from build123d import *

# Parameters (mm, degrees)
F1_DEPTH       = 40
F3_D           = 6.6
F3_CSINK_D     = 13.44
F3_CSINK_ANGLE = 90


# Not quite as in the source:
# - a feature names something its author has since deleted; it is built from what else it names


with BuildPart() as f1:
    # F0 (on Front) → F1 (new body)
    with BuildSketch(Plane.XZ):
        Polygon((52.3067873225, 0), (0, 0), (0, -17), align=None)
    extrude(amount=F1_DEPTH)

    # F3 (through all)
    with Locations(Plane(origin=(4.997243483, 0, -15.3758677686), x_dir=(0.9510324968, 0, 0.3090909091), z_dir=(0.3090909091, 0, -0.9510324968))):
        with Locations((9.5479916781, 20), (30.6618269533, 20)):
            CounterSinkHole(F3_D / 2, F3_CSINK_D / 2, counter_sink_angle=F3_CSINK_ANGLE)


solid = f1.part
The model under review builds one solid part; all positions refer to its coordinate system, in mm. Give positions to 0.01 mm unless a question says otherwise; leave off trailing zeros. Order: outer loops, then holes, each group sorted by start corner. A loop starts at its lowest first (then second) coordinate and runs counter-clockwise, first axis right, second up. Notation, with made-up numbers: M 24,62.25 L 58,62.25 A11 cw 58,70.25 Z; hole C 61.25,56 d2. An arc over 180 degrees is marked long. Answer in a Markdown table with one row per item. Add a question column.
1. Add section B-B on y = -21. Count the separate pieces of the cut face and the enclosed holes in it, plus the area to 3 significant figures.
2. Add section D-D on x = 4. State the section outline as (y, z) points.
3. Add section C-C on z = -15.75. State the section outline as (x, y) points, plus the area to 3 significant figures.
4. Mouldability with a two-part tool opening along Y and no side actions: class faces 1 (the conical face through (16.37, -20.15, -8.26)), 2 (the flat face through (20, -40, -6)), 3 (the cylindrical face through (8.35, -20.99, -4.98)), 4 (the flat face through (25.79, -19.72, -8.62)) as released by +Y, released by -Y, zero draft, split by the parting line, or undercut.
5. For pin 1 Ø8 at (x, y) = (32, -13) entering from -Z; pin 2 Ø10 at (x, z) = (37.5, -13.5) entering from -Y, all flat-tipped, find the tip position at first contact; note any pin that passes through.
6. To check wall thickness, follow line 1 along Y through (x, z) = (30.5, -3); line 2 along X through (y, z) = (-19, -5.75); line 3 along X through (y, z) = (-19, -5). State the ranges of each line that lie inside material, in increasing order.
7. Add section A-A on y = -8.5. State the section outline as (x, z) points, plus the area to 3 significant figures.
The answers:
| question | item | result |
|---|---|---|
| 1 | separate pieces | 3 |
| 1 | enclosed holes | 0 |
| 1 | area | 299 mm2 |
| 2 | outline | M -40,-15.7 L 0,-15.7 L 0,0 L -40,0 Z |
| 3 | outline | M 0,-40 L 3.85,-40 L 3.85,0 L 0,0 Z |
| 3 | area | 154 mm2 |
| 4 | face 1 | undercut |
| 4 | face 2 | released by -Y |
| 4 | face 3 | undercut |
| 4 | face 4 | zero draft |
| 5 | pin 1 | z = -7.9 |
| 5 | pin 2 | through |
| 6 | line 1 | -40 to -22.05, -17.95 to 0 |
| 6 | line 2 | 0 to 8.6, 15.22 to 28.98 |
| 6 | line 3 | 0 to 8.36, 14.97 to 29.37 |
| 7 | outline | M 0,-17 L 52.31,0 L 0,0 Z |
| 7 | area | 445 mm2 |
